from build123d import *

# Parameters (mm, degrees)
F0_R      = 6.369353
F0_R_2    = 5.980064
F0_R_3    = 5.586292
F0_R_4    = 6.448317
F1_DEPTH  = 24.13
F2_W      = 13.556814
F2_H      = 8.429615
F3_DEPTH  = 37.846
F4_W      = 13.355822
F4_H      = 12.236101
F5_DEPTH  = 46.736
F6_R      = 11.43
F7_DEPTH  = 53.594
F8_R      = 11.43
F9_DEPTH  = 57.404
F10_W     = 85.677572
F10_H     = 10.745444
F11_DEPTH = 11.684


with BuildPart() as f1:
    # F0 (on Top) → F1 (new body)
    with BuildSketch(Plane.XY):
        with BuildLine():
            ThreePointArc((-37.110602, 26.470889), (-41.57278, 24.595866), (-43.417405, 20.121036))
            Line((-43.417405, 20.121036), (-43.417405, -22.982161))
            ThreePointArc((-43.417405, -22.982161), (-41.557533, -27.472289), (-37.067405, -29.332161))
            Line((-37.067405, -29.332161), (35.615317, -29.332161))
            ThreePointArc((35.615317, -29.332161), (40.105445, -27.472289), (41.965317, -22.982161))
            Line((41.965317, -22.982161), (41.965317, 20.615476))
            ThreePointArc((41.965317, 20.615476), (40.090147, 25.120851), (35.572121, 26.965329))
            Line((35.572121, 26.965329), (-37.110602, 26.470889))
        make_face()
        with Locations((-31.80071, -20.038802)):
            Circle(F0_R, mode=Mode.SUBTRACT)
        with Locations((30.058201, -20.038802)):
            Circle(F0_R_2, mode=Mode.SUBTRACT)
        with Locations((-31.80071, 17.715463)):
            Circle(F0_R_3, mode=Mode.SUBTRACT)
        with Locations((31.21987, 17.715463)):
            Circle(F0_R_4, mode=Mode.SUBTRACT)
    extrude(amount=F1_DEPTH)

    # F2 (on Front) → F3 (cut)
    with BuildSketch(Plane.XZ):
        with Locations((0.043029, 21.780576)):
            Rectangle(F2_W, F2_H)
    extrude(amount=-F3_DEPTH, mode=Mode.SUBTRACT)

    # F4 (on Front) → F5 (cut)
    with BuildSketch(Plane.XZ):
        with Locations((0.143518, 23.694851)):
            Rectangle(F4_W, F4_H)
    extrude(amount=F5_DEPTH, mode=Mode.SUBTRACT)

    # F6 (on Right) → F7 (cut)
    with BuildSketch(Plane.YZ):
        with Locations((0.145212, 24.395064)):
            Circle(F6_R)
    extrude(amount=-F7_DEPTH, mode=Mode.SUBTRACT)

    # F8 (on Right) → F9 (cut)
    with BuildSketch(Plane.YZ):
        with Locations((-0.145212, 24.395064)):
            Circle(F8_R)
    extrude(amount=F9_DEPTH, mode=Mode.SUBTRACT)

    # F10 (on Top) → F11 (join)
    with BuildSketch(Plane.XY):
        with Locations((-0.578619, -1.016461)):
            Rectangle(F10_W, F10_H)
    extrude(amount=-F11_DEPTH)


solid = f1.part
Model file for the job. Use its own axes, mm. A direction names the side the tool comes from. Give positions to 0.01 mm unless a question says otherwise; leave off trailing zeros. Write each loop counter-clockwise with the first axis right and the second up, starting at its lowest first coordinate (ties: lowest second). Pieces come first, ordered by that corner, then holes. Notation, with made-up numbers: M 73.5,-14.5 L 114.5,-14.5 A21 ccw 114.5,2.5 Z; hole C 3,-21.5 d7. An arc over 180 degrees is marked long. One line per item, written item: value. Start each with the question number.
Q1. Saw through at B-B, the plane y = -21. Write the cut outline in (x, z).
Q2. Drop flat-ended pins along their axis: pin 1 Ø9.5 at (x, z) = (-13, -5.5) entering from +Y; pin 2 Ø5.5 at (y, z) = (18.5, 20.5) entering from +X; pin 3 Ø25 at (x, y) = (11, -23) entering from -Z. Give the stop position or say it passes through.
Q3. Saw through at D-D, the plane x = 9.5. Write the cut outline in (y, z), plus the area to 3 significant figures.
Q4. Saw through at A-A, the plane z = 19. Write the cut outline in (x, y).
Q5. 3-axis set-ups, long thin cutter, end or side, ignore diameter. For faces 1 (the flat face through (0, -19, 17.577)), 2 (the flat face through (-1, -6.389, -6)), 3 (the cylindrical face through (20.689, -0.393, 12.968)): which of +Z, -Z, +X, -X, +Y, -Y reach the whole face in a straight line?
Q6. Probe probe 1 along X at (y, z) = (15, 14); probe 2 along Y at (x, z) = (27, 4); probe 3 along X at (y, z) = (-23, 10). List the from-to ranges inside material, lowest first. Write a range as [from, to].
Q7. Saw through at C-C, the plane z = 14. Write the cut outline in (x, y).
Output values:
1. outline: M -43.42,0 L -38.1,0 L -38.1,24.13 L -43.42,24.13 Z; M -25.5,0 L 24.16,0 L 24.16,24.13 L 6.82,24.13 L 6.82,17.58 L -6.53,17.58 L -6.53,24.13 L -25.5,24.13 Z; M 35.96,0 L 41.97,0 L 41.97,24.13 L 35.96,24.13 Z
2. pin 1: stops at y = 4.36
2. pin 2: stops at x = 41.97
2. pin 3: stops at z = 0
3. outline: M -29.33,0 L -6.39,0 L -6.39,-11.68 L 4.36,-11.68 L 4.36,0 L 26.79,0 L 26.79,24.13 L 11.28,24.13 A11.43 cw -11.57,24.13 L -29.33,24.13 Z
3. area: 1,280 mm²
4. outline: M -43.42,-22.98 A6.35 ccw -37.07,-29.33 L -6.53,-29.33 L -6.53,-9.93 L -43.42,-9.93 Z; M -43.42,10.22 L -6.74,10.22 L -6.74,26.68 L -37.11,26.47 A6.35 ccw -43.42,20.12 Z; M 6.82,-29.33 L 35.62,-29.33 A6.35 ccw 41.97,-22.98 L 41.97,-10.22 L 6.82,-10.22 Z; M 6.82,9.93 L 41.97,9.93 L 41.97,20.62 A6.35 ccw 35.57,26.97 L 6.82,26.77 Z; hole C -31.8,-20.04 d12.74; hole C -31.8,17.72 d11.17; hole C 30.06,-20.04 d11.96; hole C 31.22,17.72 d12.9
5. face 1: +Z, +Y, -Y
5. face 2: -Z, +X, -X, -Y
5. face 3: +Z, +X
6. probe 1: x = [-43.42, -36.68], [-26.92, 25.37], [37.07, 41.97]
6. probe 2: y = [-29.33, -25.18], [-14.9, 12.84], [22.59, 26.91]
6. probe 3: x = [-43.42, -37.44], [-26.16, 24.86], [35.25, 41.97]
7. outline: M -43.42,-22.98 A6.35 ccw -37.07,-29.33 L 35.62,-29.33 A6.35 ccw 41.97,-22.98 L 41.97,-4.9 L 0,-4.9 L 0,-4.61 L -43.42,-4.61 Z; M -43.42,4.9 L 0,4.9 L 0,4.61 L 41.97,4.61 L 41.97,20.62 A6.35 ccw 35.57,26.97 L -37.11,26.47 A6.35 ccw -43.42,20.12 Z; hole C -31.8,-20.04 d12.74; hole C -31.8,17.72 d11.17; hole C 30.06,-20.04 d11.96; hole C 31.22,17.72 d12.9
